Geometry: final body of the model. Coordinates: model frame, mm. A direction names the side the tool comes from. Give positions to 0.01 mm unless a question says otherwise; leave off trailing zeros. Loops run counter-clockwise (first coordinate to the right, second up) from the corner with the lowest first, then second, coordinate; pieces in that order, holes last. Notation, with made-up numbers: (34.25, -5.5) -> (42.25, -5.5) arc R20 cw to (42.25, 16.5) -> close; hole circle Ø11 at (-37, 68). An arc over 180 degrees is marked (long way). One line per item, written item: value. Start each with the question number.
Autodesk Inventor part; units mm, degrees
ref_plane "YZ Plane" through (0, 0, 0) normal (1, 0, 0) x (0, 1, 0)
ref_plane "XZ Plane" through (0, 0, 0) normal (0, 1, 0) x (-1, 0, 0)
ref_plane "XY Plane" through (0, 0, 0) normal (0, 0, 1) x (1, 0, 0)
sketch "Sketch2" plane through (0, 0, 0) normal (0, 1, 0) x (-1, 0, 0)
  line L0 (-7, 3.85) -> (-10.8, 3.85)
  line L1 (-12.8, 12.8) -> (-12.8, 9.8)
  line L2 (-10.8, 2.35) -> (-10.8, 3.85)
  line L3 (0, 0) -> (0, 7) construction
  line L4 (-12.8, 2.35) -> (-10.8, 2.35)
  line L5 (-7, 3.85) -> (-7, 0)
  line L6 (-7, 0) -> (0, 0) construction
  line L7 (-12.8, 9.8) -> (-15.8, 9.8)
  line L8 (-15.8, 9.8) -> (-15.8, 6.8)
  line L9 (-15.8, 6.8) -> (-12.8, 6.8)
  line L10 (-12.8, 6.8) -> (-12.8, 2.35)
  line L11 (-12.8, 12.8) -> (-9.8, 12.8)
  line L12 (-9.8, 12.8) -> (-9.8, 15.8)
  line L13 (-9.8, 15.8) -> (-6.8, 15.8)
  line L14 (-6.8, 15.8) -> (-6.8, 12.8)
  line L15 (0, 7) -> (-3.85, 7)
  line L16 (-3.85, 7) -> (-3.85, 10.8)
  line L17 (-3.85, 10.8) -> (-2.35, 10.8)
  line L18 (-2.35, 10.8) -> (-2.35, 12.8)
  line L19 (-2.35, 12.8) -> (-6.8, 12.8)
  line L20 (-7, -3.85) -> (-10.8, -3.85)
  line L21 (-12.8, -12.8) -> (-12.8, -9.8)
  line L22 (-10.8, -2.35) -> (-10.8, -3.85)
  line L23 (0, 0) -> (0, -7) construction
  line L24 (-12.8, -2.35) -> (-10.8, -2.35)
  line L25 (-7, -3.85) -> (-7, 0)
  line L26 (-12.8, -9.8) -> (-15.8, -9.8)
  line L27 (-15.8, -9.8) -> (-15.8, -6.8)
  line L28 (-15.8, -6.8) -> (-12.8, -6.8)
  line L29 (-12.8, -6.8) -> (-12.8, -2.35)
  line L30 (-12.8, -12.8) -> (-9.8, -12.8)
  line L31 (-9.8, -12.8) -> (-9.8, -15.8)
  line L32 (-9.8, -15.8) -> (-6.8, -15.8)
  line L33 (-6.8, -15.8) -> (-6.8, -12.8)
  line L34 (0, -7) -> (-3.85, -7)
  line L35 (-3.85, -7) -> (-3.85, -10.8)
  line L36 (-3.85, -10.8) -> (-2.35, -10.8)
  line L37 (-2.35, -10.8) -> (-2.35, -12.8)
  line L38 (-2.35, -12.8) -> (-6.8, -12.8)
  line L39 (7, 3.85) -> (10.8, 3.85)
  line L40 (12.8, 12.8) -> (12.8, 9.8)
  line L41 (10.8, 2.35) -> (10.8, 3.85)
  line L42 (12.8, 2.35) -> (10.8, 2.35)
  line L43 (7, 3.85) -> (7, 0)
  line L44 (7, 0) -> (0, 0) construction
  line L45 (12.8, 9.8) -> (15.8, 9.8)
  line L46 (15.8, 9.8) -> (15.8, 6.8)
  line L47 (15.8, 6.8) -> (12.8, 6.8)
  line L48 (12.8, 6.8) -> (12.8, 2.35)
  line L49 (12.8, 12.8) -> (9.8, 12.8)
  line L50 (9.8, 12.8) -> (9.8, 15.8)
  line L51 (9.8, 15.8) -> (6.8, 15.8)
  line L52 (6.8, 15.8) -> (6.8, 12.8)
  line L53 (0, 7) -> (3.85, 7)
  line L54 (3.85, 7) -> (3.85, 10.8)
  line L55 (3.85, 10.8) -> (2.35, 10.8)
  line L56 (2.35, 10.8) -> (2.35, 12.8)
  line L57 (2.35, 12.8) -> (6.8, 12.8)
  line L58 (7, -3.85) -> (10.8, -3.85)
  line L59 (3.85, -7) -> (3.85, -10.8)
  line L60 (2.35, -10.8) -> (2.35, -12.8)
  line L61 (3.85, -10.8) -> (2.35, -10.8)
  line L62 (7, -3.85) -> (7, 0)
  line L63 (0, -7) -> (3.85, -7)
  line L64 (2.35, -12.8) -> (6.8, -12.8)
  line L65 (9.8, -15.8) -> (6.8, -15.8)
  line L66 (6.8, -15.8) -> (6.8, -12.8)
  line L67 (9.8, -12.8) -> (9.8, -15.8)
  line L68 (12.8, -12.8) -> (9.8, -12.8)
  line L69 (12.8, -12.8) -> (12.8, -9.8)
  line L70 (10.8, -2.35) -> (10.8, -3.85)
  line L71 (12.8, -2.35) -> (10.8, -2.35)
  line L72 (12.8, -6.8) -> (12.8, -2.35)
  line L73 (12.8, -9.8) -> (15.8, -9.8)
  line L74 (15.8, -9.8) -> (15.8, -6.8)
  line L75 (15.8, -6.8) -> (12.8, -6.8)
  dimension "d4" = 2
  dimension "d8" = 3
  dimension "d9" = 3
  dimension "d11" = 3.8
  dimension "d13" = 3
  dimension "d14" = 3
  dimension "d15" = 3
  dimension "d16" = 3.85
  dimension "d17" = 3.85
  dimension "d18" = 3.8
  dimension "d20" = 2
  dimension "d22" = 3
  dimension "d23" = 3
  dimension "d27" = 2.35
  dimension "d28" = 2.35
  dimension "d29" = 7
  dimension "d30" = 7
extrude "Extrusion1" add sketch "Sketch2" along normal mid plane 6
properties part number "plunger_handle_center"
Item 1: Section C-C, the plane x = -3. Output: boundary loops of the cut face in (y, z), then the cut area to 3 significant figures.
Item 2: Mould query, pull axis X, two halves, no side actions, for faces 6 (the face through (-3.85, 0, 9)), 7 (the face through (12, 0, 2.35)), 8 (the face through (10.8, 0, 3)), 9 (the face through (15.8, 0, 8)). Classes: pulls with the +X half, pulls with the -X half, needs draft (parallel to the pull), parting line crosses it, or undercut.
Item 3: Section B-B, the plane x = 7.5. Output: boundary loops of the cut face in (y, z).
Item 4: Access query for faces 1 (the face through (2.35, 0, 12)), 2 (the face through (12.8, 0, 11)), 3 (the face through (-12.8, 0, 5)), 4 (the face through (-9.8, 0, -14)), 5 (the face through (-7, 0, 0)). Directions: +Z, -Z, +X, -X, +Y, -Y. A direction counts if a zero-diameter tool reaches every point of the face in a straight line with its end or side. Return the directions, or none.
Item 5: Pin query (flat end, axial travel): pin 1 (1.5 mm diameter, centred on y = 0, z = 2.5, fed in from +X); pin 2 (1.6 mm diameter, centred on y = 0.5, z = -11.5, fed in from -X); pin 3 (3 mm diameter, centred on x = -1, y = -0.5, fed in from +Z). Return the tip coordinate at first contact, or that it passes through.
Item 6: Ray query, line 1 along Z through (x, y) = (-13.5, 1.15); line 2 along X through (y, z) = (0.9, 12); line 3 along Z through (x, y) = (2.5, -0.35). Return the intervals inside material, ascending. Write a range as [from, to].
Item 7: Section A-A, the plane z = -9. Output: boundary loops of the cut face in (x, y), then the cut area to 3 significant figures.
Geometry check:
1. outline: (-3, -12.8) -> (3, -12.8) -> (3, -10.8) -> (-3, -10.8) -> close; (-3, -7) -> (3, -7) -> (3, 7) -> (-3, 7) -> close; (-3, 10.8) -> (3, 10.8) -> (3, 12.8) -> (-3, 12.8) -> close
1. area: 108 mm2
2. face 6: undercut
2. face 7: needs draft
2. face 8: undercut
2. face 9: pulls with the +X half
3. outline: (-3, -15.8) -> (3, -15.8) -> (3, -3.85) -> (-3, -3.85) -> close; (-3, 3.85) -> (3, 3.85) -> (3, 15.8) -> (-3, 15.8) -> close
4. face 1: +Z, +Y, -Y
4. face 2: +Z, +X, +Y, -Y
4. face 3: -X, +Y, -Y
4. face 4: -Z, -X, +Y, -Y
4. face 5: +Y, -Y
5. pin 1: stops at x = 12.8
5. pin 2: stops at x = -12.8
5. pin 3: stops at z = 12.8
6. line 1: z = [-9.8, -6.8], [6.8, 9.8]
6. line 2: x = [-12.8, -2.35], [2.35, 12.8]
6. line 3: z = [-12.8, -10.8], [-7, 7], [10.8, 12.8]
7. outline: (-15.8, -3) -> (-3.85, -3) -> (-3.85, 3) -> (-15.8, 3) -> close; (3.85, -3) -> (15.8, -3) -> (15.8, 3) -> (3.85, 3) -> close
7. area: 143 mm2
